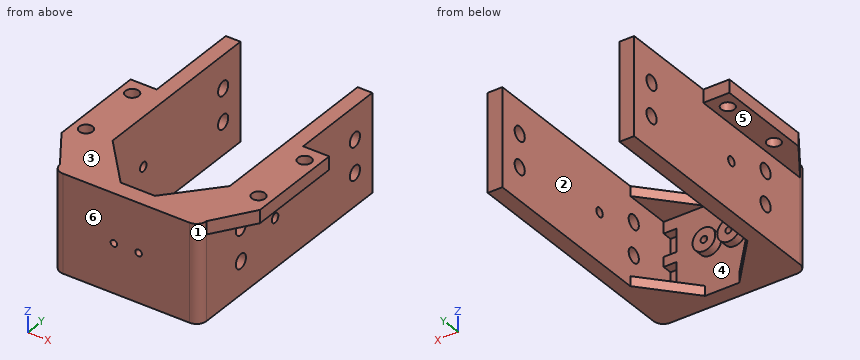
```python
from build123d import *

# Parameters (mm, degrees)
SKETCH1_W           = 45
SKETCH1_H           = 30
SKETCH1_R           = 3.5
BOSS_EXTRUDE1_DEPTH = 5
SKETCH1_4_R         = 3.5
SKETCH1_4_R_2       = 1
BOSS_EXTRUDE2_DEPTH = 7.6
SKETCH2_W           = 4.5
SKETCH2_H           = 30
BOSS_EXTRUDE3_DEPTH = 70
SKETCH3_R           = 1.4
SKETCH3_R_2         = 2.2
CUT_EXTRUDE1_DEPTH  = 4.5
FILLET1_R           = 3
SKETCH6_W           = 4.008200323
SKETCH6_H           = 7
CUT_EXTRUDE3_DEPTH  = 3
BOSS_EXTRUDE4_DEPTH = 3
SKETCH8_R           = 2.05
BOSS_EXTRUDE5_DEPTH = 4


with BuildPart() as part:
    # Sketch1 → Boss-Extrude1 (new body)
    with BuildSketch(Plane(origin=(0, 0, 0), x_dir=(1, 0, 0), z_dir=(0, 1, 0))):
        Rectangle(SKETCH1_W, SKETCH1_H)
        with Locations((3.8, 0)):
            Circle(SKETCH1_R, mode=Mode.SUBTRACT)
        with Locations((-3.8, 0)):
            Circle(SKETCH1_R, mode=Mode.SUBTRACT)
    extrude(amount=BOSS_EXTRUDE1_DEPTH)

    # Sketch1_4 → Boss-Extrude2 (add)
    with BuildSketch(Plane(origin=(0, 0, 0), x_dir=(1, 0, 0), z_dir=(0, 1, 0))):
        with Locations((3.8, 0)):
            Circle(SKETCH1_4_R)
        with Locations((3.8, 0)):
            Circle(SKETCH1_4_R_2, mode=Mode.SUBTRACT)
        with Locations((-3.8, 0)):
            Circle(SKETCH1_4_R)
        with Locations((-3.8, 0)):
            Circle(SKETCH1_4_R_2, mode=Mode.SUBTRACT)
    extrude(amount=BOSS_EXTRUDE2_DEPTH)

    # Sketch2 → Boss-Extrude3 (add)
    with BuildSketch(Plane(origin=(0, 5, 0), x_dir=(1, 0, 0), z_dir=(0, 1, 0))):
        with Locations((-20.25, 0)):
            Rectangle(SKETCH2_W, SKETCH2_H)
        with Locations((20.25, 0)):
            Rectangle(SKETCH2_W, SKETCH2_H)
    extrude(amount=BOSS_EXTRUDE3_DEPTH)

    # Sketch3 → Cut-Extrude1 (cut)
    with BuildSketch(Plane.ZY.offset(22.5)):
        with Locations((0, 32.83)):
            Circle(SKETCH3_R)
        with Locations((5, 17.98)):
            Circle(SKETCH3_R_2)
        with Locations((-5, 17.98)):
            Circle(SKETCH3_R_2)
        with Locations((-5, 67.48)):
            Circle(SKETCH3_R_2)
        with Locations((5, 67.48)):
            Circle(SKETCH3_R_2)
    cut_extrude1 = extrude(amount=-CUT_EXTRUDE1_DEPTH, mode=Mode.SUBTRACT)

    # Fillet1
    fillet1_edges = [part.edges().sort_by_distance(p)[0] for p in [
        (-22.5, 0, 0),
        (22.5, 0, 0),
    ]]
    fillet(fillet1_edges, radius=FILLET1_R)

    # Sketch6 → Cut-Extrude3 (cut)
    with BuildSketch(Plane(origin=(0, 5, 0), x_dir=(1, 0, 0), z_dir=(0, 1, 0))):
        with Locations((-15.995899839, 5)):
            Rectangle(SKETCH6_W, SKETCH6_H)
        with Locations((-15.995899839, -5)):
            Rectangle(SKETCH6_W, SKETCH6_H)
    cut_extrude3 = extrude(amount=-CUT_EXTRUDE3_DEPTH, mode=Mode.SUBTRACT)

    # Mirror1: Cut-Extrude1, Cut-Extrude3 across plane
    add(cut_extrude1.mirror(Plane(origin=(0, 0, 0), x_dir=(0, 0, 1), z_dir=(1, 0, 0))), mode=Mode.SUBTRACT)
    add(cut_extrude3.mirror(Plane(origin=(0, 0, 0), x_dir=(0, 0, 1), z_dir=(1, 0, 0))), mode=Mode.SUBTRACT)

    # Sketch7 → Boss-Extrude4 (add)
    with BuildSketch(Plane.XY.offset(15)):
        Polygon((-18, 19.5), (-5.259164302, 5), (-18, 5), align=None)
        Polygon((5.26, 5), (18, 5), (18, 19.5), align=None)
    boss_extrude4 = extrude(amount=-BOSS_EXTRUDE4_DEPTH)

    # Mirror2: Boss-Extrude4 across plane
    add(boss_extrude4.mirror(Plane.XY))

    # Sketch8 → Boss-Extrude5 (add)
    with BuildSketch(Plane.XY.offset(15)):
        Polygon((-22.5, 15), (-22.5, 45), (-30.5, 45), (-30.5, 15), (-22.5, 3), align=None)
        with Locations((-26.5, 40)):
            Circle(SKETCH8_R, mode=Mode.SUBTRACT)
        with Locations((-26.5, 20)):
            Circle(SKETCH8_R, mode=Mode.SUBTRACT)
        Polygon((30.5, 15), (22.5, 3), (22.5, 15), (22.5, 45), (30.5, 45), align=None)
        with Locations((26.5, 20)):
            Circle(SKETCH8_R, mode=Mode.SUBTRACT)
        with Locations((26.5, 40)):
            Circle(SKETCH8_R, mode=Mode.SUBTRACT)
    extrude(amount=-BOSS_EXTRUDE5_DEPTH)


solid = part.part
```
Part model, mm, in its own coordinate system. Face numbers are marked on the shaded views. A direction names the side the tool comes from. Give positions to 0.01 mm unless a question says otherwise; leave off trailing zeros. Order: outer loops, then holes, each group sorted by start corner. A loop starts at its lowest first (then second) coordinate and runs counter-clockwise, first axis right, second up. Notation, with made-up numbers: M 13,60.5 L 51,60.5 A13 cw 51,75.5 Z; hole C 22.25,44 d9. An arc over 180 degrees is marked long. Use a Markdown table: item, result. Add a question column.
(1) Mould opens along X. For the marked faces 1, 2 and 3 say: +X half, -X half, draft (parallel to the pull), parting line (faces both ways), or undercut.
(2) Probe line 1 along X through (y, z) = (69, 1.5); line 2 along Z through (x, y) = (-3.8, 3.5); line 3 along Z through (x, y) = (25.5, 27). List the from-to ranges inside material, lowest first. Write a range as [from, to].
(3) Saw through at A-A, the plane x = 3.8. Give the cut face in (y, z).
(4) Drop flat-ended pins along their axis: P1, Ø1, axis at y = 14, z = 8, coming from the -X side; P2, Ø5.5, axis at x = -3, z = 1, coming from the +Y side; P3, Ø15, axis at y = 46, z = 3.5, coming from the +X side; P4, Ø5, axis at x = 15, y = 22.5, coming from the -Z side. Give the stop position or say it passes through.
(5) 3-axis set-ups, long thin cutter, end or side, ignore diameter. For the marked faces 4, 5 and 6: which of +Z, -Z, +X, -X, +Y, -Y reach the whole face in a straight line?
(6) Saw through at B-B, the plane y = 61. Give the cut face in (x, z).
(7) Saw through at C-C, the plane z = 5. Give the number of separate pieces and of enclosed holes in the cut face, and give its area (3 significant figures).
(8) Saw through at D-D, the plane x = -26.5. Give the cut face in (y, z), and give its area (3 significant figures).
Answer key:
| question | item | result |
|---|---|---|
| 1 | face 1 | +X half |
| 1 | face 2 | undercut |
| 1 | face 3 | draft |
| 2 | line 1 | [-22.5, -18], [18, 22.5] |
| 2 | line 2 | [-15, -1], [1, 15] |
| 2 | line 3 | [11, 15] |
| 3 | outline | M 0,-15 L 5,-15 L 5,-3.5 L 7.6,-3.5 L 7.6,-1 L 0,-1 Z; M 0,1 L 7.6,1 L 7.6,3.5 L 5,3.5 L 5,15 L 0,15 Z |
| 4 | P1 | x = -22.5 |
| 4 | P2 | y = 7.6 |
| 4 | P3 | x = 22.5 |
| 4 | P4 | through |
| 5 | face 4 | +Y |
| 5 | face 5 | -Z, -X, +Y, -Y |
| 5 | face 6 | +Z, -Z, +X, -X, -Y |
| 6 | outline | M -22.5,-15 L -18,-15 L -18,15 L -22.5,15 Z; M 18,-15 L 22.5,-15 L 22.5,15 L 18,15 Z |
| 7 | separate pieces | 5 |
| 7 | enclosed holes | 0 |
| 7 | area | 748 mm^2 |
| 8 | outline | M 9,11 L 17.95,11 L 17.95,15 L 9,15 Z; M 22.05,11 L 37.95,11 L 37.95,15 L 22.05,15 Z; M 42.05,11 L 45,11 L 45,15 L 42.05,15 Z |
| 8 | area | 111 mm^2 |
